CAD build for the part. Positions are in the model's coordinates, mm. Face numbers are marked on the shaded views. A direction names the side the tool comes from. Round coordinates to 2 decimals unless told otherwise and drop trailing zeros. Loops run counter-clockwise (first coordinate to the right, second up) from the corner with the lowest first, then second, coordinate; pieces in that order, holes last. Notation, with made-up numbers: (60.25, -31.5) - (106.25, -31.5) arc R13 ccw to (106.25, -8.5) - close; hole circle Ø11 at (84, 33). An arc over 180 degrees is marked (long way). One line per question, with ' | ' between items.
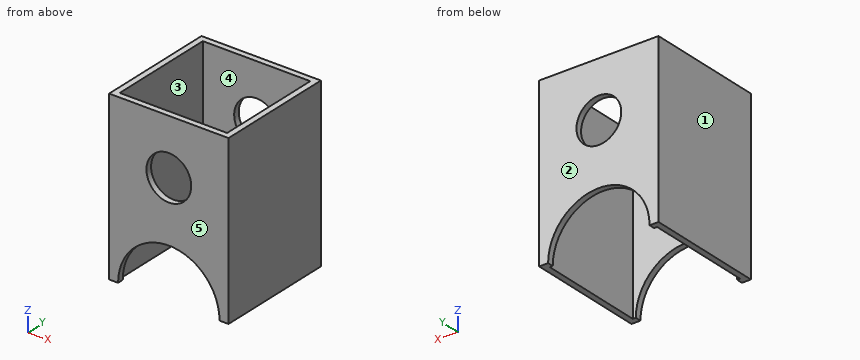
Autodesk Inventor part; units mm, degrees
ref_plane "YZ Plane" through (0, 0, 0) normal (1, 0, 0) x (0, 1, 0)
ref_plane "XZ Plane" through (0, 0, 0) normal (0, 1, 0) x (-1, 0, 0)
ref_plane "XY Plane" through (0, 0, 0) normal (0, 0, 1) x (1, 0, 0)
sketch "スケッチ1" plane through (0, 0, 0) normal (0, 0, 1) x (1, 0, 0)
  line L0 (-16, -16) -> (16, -16)
  line L1 (16, -16) -> (16, 16)
  line L2 (16, 16) -> (-16, 16)
  line L3 (-16, 16) -> (-16, -16)
  line L4 (-16, -16) -> (16, 16) construction
  line L5 (16, -16) -> (-16, 16) construction
  line L6 (-14.4, 14.4) -> (14.4, 14.4)
  line L7 (14.4, 14.4) -> (14.4, -14.4)
  line L8 (14.4, -14.4) -> (-14.4, -14.4)
  line L9 (-14.4, -14.4) -> (-14.4, 14.4)
  point P0 (0, 0)
  dimension "d0" = 32
  dimension "d1" = 32
  dimension "d2" = 1.6
extrude "押し出し1" add sketch "スケッチ1" along normal blind 45
sketch "スケッチ2" plane through (-16, 16, 0) normal (0, 1, 0) x (1, 0, 0)
  circle A0 centre (16, 0) radius 13.6
  dimension "d5" = 27.2
extrude "押し出し2" cut sketch "スケッチ2" against normal blind 32
sketch "スケッチ3" plane through (-16, 16, 45) normal (0, 1, 0) x (1, 0, 0)
  line L0 (32, 0) -> (0, 0)
  point P0 (16, 45)
  point P1 (16, 15)
  dimension "d16" = 30
hole "穴1" at (0, 16, 30) direction (0, -1, 0) diameter 12 end through all
sketch "スケッチ4" plane through (-16, 16, 45) normal (0, 1, 0) x (1, 0, 0)
  circle A0 centre (16, 15) radius 13.6
  point P0 (16, 45)
  dimension "d17" = 30
  dimension "d18" = 27.2
properties part number "軸受上用"
(1) Cut at A-A, the plane z = 30. Write the cut outline in (x, y).
Results found:
outline: (-16, -16) - (-6, -16) - (-6, -14.4) - (-14.4, -14.4) - (-14.4, 14.4) - (-6, 14.4) - (-6, 16) - (-16, 16) - close; (6, -16) - (16, -16) - (16, 16) - (6, 16) - (6, 14.4) - (14.4, 14.4) - (14.4, -14.4) - (6, -14.4) - close
(2) Tool access for the marked faces 4 and 5: list every direction of +Z, -Z, +X, -X, +Y, -Y with a clear straight run to the whole face (end or side of a thin tool).
Results found:
face 4: +Z, -Z | face 5: +Z, -Z, +X, -X, -Y
(3) Two-plate mould, pull along X, no slides. Class the marked faces 1, 2 and 3: released by +X, released by -X, zero draft, split by the parting line, or undercut.
Results found:
face 1: released by -X | face 2: zero draft | face 3: undercut
(4) Cut at C-C, the plane x = 0. Write the cut outline in (y, z), then the cut area to 3 significant figures.
Results found:
outline: (-16, 13.6) - (-14.4, 13.6) - (-14.4, 24) - (-16, 24) - close; (-16, 36) - (-14.4, 36) - (-14.4, 45) - (-16, 45) - close; (14.4, 13.6) - (16, 13.6) - (16, 24) - (14.4, 24) - close; (14.4, 36) - (16, 36) - (16, 45) - (14.4, 45) - close | area: 62.1 mm²
(5) Cut at D-D, the plane z = 41.5. Write the cut outline in (x, y).
Results found:
outline: (-16, -16) - (16, -16) - (16, 16) - (-16, 16) - close; hole (-14.4, -14.4) - (14.4, -14.4) - (14.4, 14.4) - (-14.4, 14.4) - close
(6) Probe L1, parallel to X at y = 13.5, z = 8.5; L2, parallel to Z at x = 0, y = 14.8. List the from-to ranges inside material, lowest first.
Results found:
L1: x = -16 to -14.4, 14.4 to 16 | L2: z = 13.6 to 24, 36 to 45
(7) Cut at B-B, the plane y = -11.5. Write the cut outline in (x, z).
Results found:
outline: (-16, 0) - (-14.4, 0) - (-14.4, 45) - (-16, 45) - close; (14.4, 0) - (16, 0) - (16, 45) - (14.4, 45) - close
